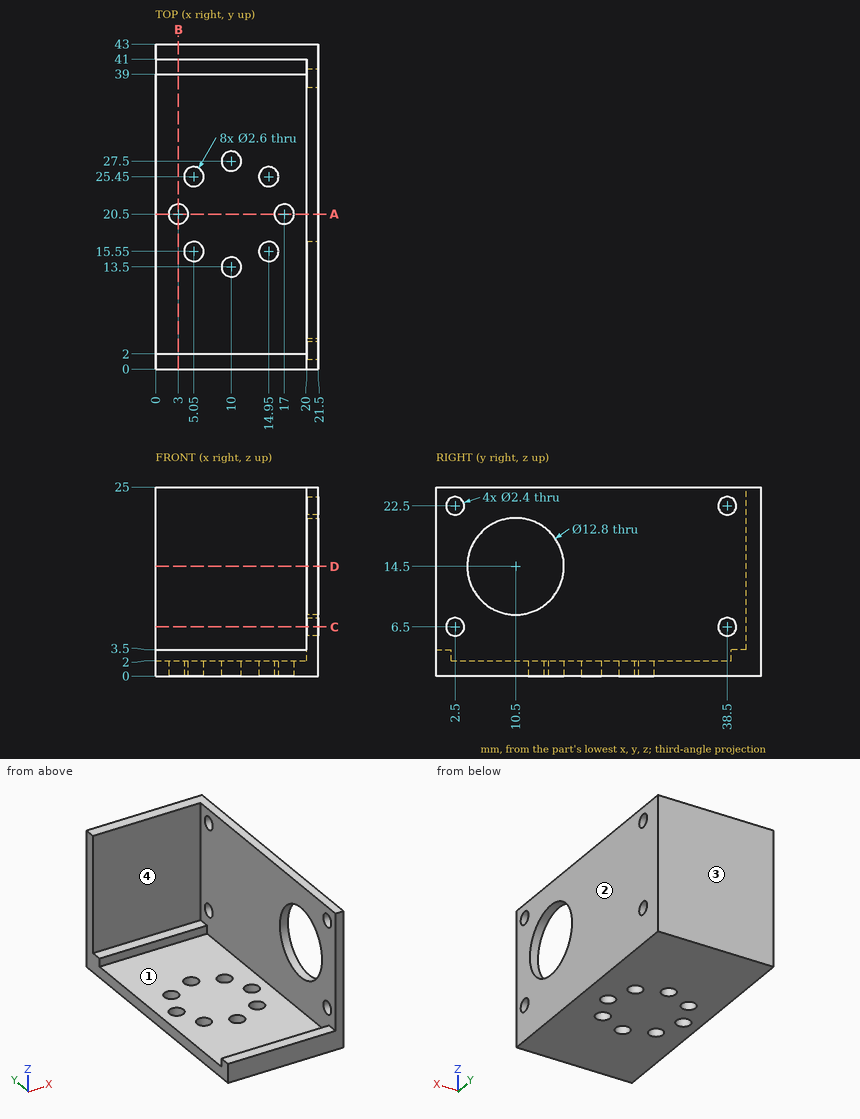
Could you check a few things on this drawing? It's one solid part, dimensions in mm from its lowest x, y, z. Give positions to 0.01 mm unless a question says otherwise; leave off trailing zeros. Order: outer loops, then holes, each group sorted by start corner. A loop starts at its lowest first (then second) coordinate and runs counter-clockwise, first axis right, second up. Notation, with made-up numbers: (23, -27.5) - (54, -27.5) arc R13 ccw to (54, -22.5) - close; hole circle Ø1 at (44.5, -40). An arc over 180 degrees is marked (long way). One line per question, with ' | ' between items. Start each with the question number.
Item 1: I need wall thicknesses on probe 1 along Y at (x, z) = (20.65, 22.5); probe 2 along Y at (x, z) = (8.25, 11.5); probe 3 along X at (y, z) = (19, 5.75). Which ranges of each line are inside material? Lowest first, please. Write a range as [from, to].
Item 2: I want a section at C-C on z = 6.5. Write out the boundary of the cut face in (x, y).
Item 3: I want a section at A-A on y = 20.5. Write out the boundary of the cut face in (x, z).
Item 4: I'm going to push flat-ended pins straight in: pin 1 Ø0.8 at (x, z) = (9.5, 3) entering from -Y; pin 2 Ø2 at (y, z) = (23, 3.5) entering from -X; pin 3 Ø5 at (x, z) = (16.5, 13.5) entering from -Y; pin 4 Ø3.5 at (x, y) = (10, 27.5) entering from +Z. Where does each tip first touch, or does it pass through?
Item 5: I want a section at D-D on z = 14.5. Write out the boundary of the cut face in (x, y).
Item 6: I want a section at B-B on x = 3. Write out the boundary of the cut face in (y, z), then the cut area to 3 significant figures.
Item 7: Thinking about a two-plate mould opening in Y: for the marked faces 1, 2, 3 and 4, which applies, pulls with the +Y half, pulls with the -Y half, needs draft (parallel to the pull), parting line crosses it, or undercut?
Verdict:
1) probe 1: [0, 1.3], [3.7, 37.3], [39.7, 43] | probe 2: [41, 43] | probe 3: [20, 21.5]
2) outline: (0, 41) - (20, 41) - (20, 39.7) - (21.5, 39.7) - (21.5, 43) - (0, 43) - close; (20, 0) - (21.5, 0) - (21.5, 1.3) - (20, 1.3) - close; (20, 3.7) - (21.5, 3.7) - (21.5, 37.3) - (20, 37.3) - close
3) outline: (0, 0) - (1.7, 0) - (1.7, 2) - (0, 2) - close; (4.3, 0) - (15.7, 0) - (15.7, 2) - (4.3, 2) - close; (18.3, 0) - (21.5, 0) - (21.5, 25) - (20, 25) - (20, 2) - (18.3, 2) - close
4) pin 1: y = 0 | pin 2: x = 20 | pin 3: y = 41 | pin 4: z = 2
5) outline: (0, 41) - (20, 41) - (20, 16.9) - (21.5, 16.9) - (21.5, 43) - (0, 43) - close; (20, 0) - (21.5, 0) - (21.5, 4.1) - (20, 4.1) - close
6) outline: (0, 0) - (19.2, 0) - (19.2, 2) - (2, 2) - (2, 3.5) - (0, 3.5) - close; (21.8, 0) - (43, 0) - (43, 25) - (41, 25) - (41, 3.5) - (39, 3.5) - (39, 2) - (21.8, 2) - close | area: 133 mm^2
7) face 1: undercut | face 2: needs draft | face 3: pulls with the +Y half | face 4: pulls with the -Y half
